from build123d import *

# Parameters (mm, degrees)
BOSS_EXTRUDE1_DEPTH = 80
CUT_EXTRUDE1_DEPTH  = 65
SKETCH3_R           = 3
SKETCH3_W           = 10
SKETCH3_H           = 10
BOSS_EXTRUDE2_DEPTH = 5


with BuildPart() as part:
    # Sketch1 → Boss-Extrude1 (new body)
    with BuildSketch(Plane(origin=(0, 0, 0), x_dir=(1, 0, 0), z_dir=(0, 1, 0))):
        with BuildLine():
            Line((-40, -40), (-40, -15.27864045))
            ThreePointArc((-40, -15.27864045), (-24.494897428, -114.772255751), (60, -60))
            ThreePointArc((60, -60), (54.772255751, -35.505102572), (40, -15.27864045))
            Line((40, -15.27864045), (40, -40))
            Line((40, -40), (-40, -40))
        make_face()
        with BuildLine():
            ThreePointArc((40, -15.27864045), (0, 0), (-40, -15.27864045))
            Line((-40, -15.27864045), (-40, -40))
            Line((-40, -40), (40, -40))
            Line((40, -40), (40, -15.27864045))
        make_face()
        with BuildLine():
            Line((40, 40), (-40, 40))
            Line((-40, 40), (-40, -15.27864045))
            ThreePointArc((-40, -15.27864045), (0, 0), (40, -15.27864045))
            Line((40, -15.27864045), (40, 40))
        make_face()
    extrude(amount=BOSS_EXTRUDE1_DEPTH)

    # Sketch2 → Cut-Extrude1 (cut)
    with BuildSketch(Plane(origin=(0, 80, 0), x_dir=(1, 0, 0), z_dir=(0, 1, 0))):
        with BuildLine():
            Line((30, 30), (-30, 30))
            Line((-30, 30), (-30, -20))
            ThreePointArc((-30, -20), (0, -10), (30, -20))
            Line((30, -20), (30, 30))
        make_face()
        with BuildLine():
            ThreePointArc((30, -20), (0, -10), (-30, -20))
            Line((-30, -20), (-30, -30))
            Line((-30, -30), (30, -30))
            Line((30, -30), (30, -20))
        make_face()
        with BuildLine():
            Line((-30, -30), (-30, -20))
            ThreePointArc((-30, -20), (-22.360679775, -104.72135955), (50, -60))
            ThreePointArc((50, -60), (44.72135955, -37.639320225), (30, -20))
            Line((30, -20), (30, -30))
            Line((30, -30), (-30, -30))
        make_face()
    extrude(amount=-CUT_EXTRUDE1_DEPTH, mode=Mode.SUBTRACT)

    # Sketch3 → Boss-Extrude2 (add)
    # profile 1 of 6: a face of its own
    with BuildSketch(Plane.XZ):
        with BuildLine():
            Line((-75, 52.5), (-59.529404499, 52.5))
            ThreePointArc((-59.529404499, 52.5), (-60, 60), (-59.529404499, 67.5))
            Line((-59.529404499, 67.5), (-75, 67.5))
            Line((-75, 67.5), (-75, 52.5))
        make_face()
        with Locations(Location((-67.5, 60, 0), (0, 0, 270))):
            Circle(SKETCH3_R, mode=Mode.SUBTRACT)
    # profile 2 of 6: a face of its own
    with BuildSketch(Plane.XZ):
        with BuildLine():
            ThreePointArc((59.529404499, 67.5), (60, 60), (59.529404499, 52.5))
            Line((59.529404499, 52.5), (75, 52.5))
            Line((75, 52.5), (75, 67.5))
            Line((75, 67.5), (59.529404499, 67.5))
        make_face()
        with Locations(Location((67.5, 60, 0), (0, 0, 270))):
            Circle(SKETCH3_R, mode=Mode.SUBTRACT)
    # profile 3 of 6: a face of its own
    with BuildSketch(Plane.XZ):
        with Locations((-45, -35)):
            Rectangle(SKETCH3_W, SKETCH3_H)
        with Locations(Location((-45, -35, 0), (0, 0, 270))):
            Circle(SKETCH3_R, mode=Mode.SUBTRACT)
    # profile 4 of 6: a face of its own
    with BuildSketch(Plane.XZ):
        with Locations((-35, -45)):
            Rectangle(SKETCH3_W, SKETCH3_H)
        with Locations(Location((-35, -45, 0), (0, 0, 270))):
            Circle(SKETCH3_R, mode=Mode.SUBTRACT)
    # profile 5 of 6: a face of its own
    with BuildSketch(Plane.XZ):
        with Locations((35, -45)):
            Rectangle(SKETCH3_W, SKETCH3_H)
        with Locations(Location((35, -45, 0), (0, 0, 270))):
            Circle(SKETCH3_R, mode=Mode.SUBTRACT)
    # profile 6 of 6: a face of its own
    with BuildSketch(Plane.XZ):
        with Locations((45, -35)):
            Rectangle(SKETCH3_W, SKETCH3_H)
        with Locations(Location((45, -35, 0), (0, 0, 270))):
            Circle(SKETCH3_R, mode=Mode.SUBTRACT)
    extrude(amount=-BOSS_EXTRUDE2_DEPTH)


solid = part.part
The model under review builds one solid part; all positions refer to its coordinate system, in mm. A direction names the side the tool comes from. Round coordinates to 2 decimals unless told otherwise and drop trailing zeros. Write each loop counter-clockwise with the first axis right and the second up, starting at its lowest first coordinate (ties: lowest second). Pieces come first, ordered by that corner, then holes. Notation, with made-up numbers: M 14,26 L 54,26 A28 cw 54,45 Z; hole C 46,44.25 d11. An arc over 180 degrees is marked long. Use a Markdown table: item, result. Add a question column.
Q1. We need section A-A, the plane z = -45. State the section outline as (x, y) points.
Q2. We need section D-D, the plane x = 35. State the section outline as (y, z) points, plus the area to 3 significant figures.
Q3. To check wall thickness, follow line 1 (X direction, y = 2.3, z = 60); line 2 (X direction, y = 3, z = -45); line 3 (X direction, y = 76, z = 12). State the ranges of each line that lie inside material, in increasing order.
Q4. The part is to be moulded in two halves that separate along X. For faces 6 (the face through (75, 2, 60)), 7 (the face through (31, 80, 16)), 8 (the face through (30, 48, -5)), say which applies: pulls with the +X half, pulls with the -X half, needs draft (parallel to the pull), parting line crosses it, or undercut.
Q5. Insertion check: pin 1 (12 mm diameter, centred on y = 69.5, z = -4, fed in from -X); pin 2 (3 mm diameter, centred on x = 45.5, z = -33, fed in from +Y); pin 3 (12 mm diameter, centred on y = 37.5, z = 81, fed in from -X); pin 4 (5.5 mm diameter, centred on x = 35, z = -45, fed in from +Y). Each pin has a flat end and moves straight along its axis. Give the tip position at first contact, or say it passes through.
Q6. Machinability: for faces 1 (the face through (-45, 2, -30)), 2 (the face through (-1.75, 47.96, 109.97)), 3 (the face through (-67, 2, 67.5)), 4 (the face through (-32.8, 5, -42.7)), 5 (the face through (30, 2, -45)), which of the approach directions +Z, -Z, +X, -X, +Y, -Y give a long, thin tool a straight path to every point of the face, cutting with its end or side? Answer none if there is none.
Q7. We need section C-C, the plane x = -45. State the section outline as (y, z) points.
Q8. We need section B-B, the plane y = 17. State the section outline as (x, z) points.
Findings below:
| question | item | result |
|---|---|---|
| 1 | outline | M -40,0 L -38,0 L -38,5 L -40,5 Z; M -32,0 L -30,0 L -30,5 L -32,5 Z; M 30,0 L 32,0 L 32,5 L 30,5 Z; M 38,0 L 40,0 L 40,5 L 38,5 Z |
| 2 | outline | M 0,-50 L 5,-50 L 5,-48 L 0,-48 Z; M 0,-42 L 5,-42 L 5,-40 L 80,-40 L 80,24.29 L 15,24.29 L 15,95.71 L 80,95.71 L 80,108.73 L 0,108.73 Z |
| 2 | area | 7,280 mm² |
| 3 | line 1 | x = -75 to -70.5, -64.5 to 64.5, 70.5 to 75 |
| 3 | line 2 | x = -40 to -38, -32 to -30, 30 to 32, 38 to 40 |
| 3 | line 3 | x = -40 to -30, 30 to 40 |
| 4 | face 6 | pulls with the +X half |
| 4 | face 7 | needs draft |
| 4 | face 8 | undercut |
| 5 | pin 1 | stops at x = -40 |
| 5 | pin 2 | stops at y = 5 |
| 5 | pin 3 | stops at x = -58.09 |
| 5 | pin 4 | passes through |
| 6 | face 1 | -X, +Y, -Y |
| 6 | face 2 | +Y |
| 6 | face 3 | +Z, -X, +Y, -Y |
| 6 | face 4 | -Z, +X, -X, +Y |
| 6 | face 5 | -Z, +Y, -Y |
| 7 | outline | M 0,-40 L 5,-40 L 5,-38 L 0,-38 Z; M 0,-32 L 5,-32 L 5,-30 L 0,-30 Z; M 0,20.31 L 80,20.31 L 80,38.21 L 15,38.21 L 15,81.79 L 80,81.79 L 80,99.69 L 0,99.69 Z |
| 8 | outline | M -40,-40 L 40,-40 L 40,15.28 A60 ccw long -40,15.28 Z; hole M -30,-30 L 30,-30 L 30,20 A50 ccw long -30,20 Z |
